CAD build for the part. Positions are in the model's coordinates, mm. A direction names the side the tool comes from. Round coordinates to 2 decimals unless told otherwise and drop trailing zeros. Write each loop counter-clockwise with the first axis right and the second up, starting at its lowest first coordinate (ties: lowest second). Pieces come first, ordered by that corner, then holes. Notation, with made-up numbers: (37, 3) - (92, 3) arc R29 cw to (92, 30) - close; hole circle Ø7 at (-20.75, 28). An arc over 180 degrees is marked (long way). Put each result on its own line as item: value. Start each with the question number.
Item 1: Cut at A-A (x = 13). Give the cut face in (y, z).
Item 2: Cut at D-D (x = 32.9). Give the cut face in (y, z), and give its area (3 significant figures).
Item 3: 3-axis set-ups, long thin cutter, end or side, ignore diameter. For faces 1 (the cylindrical face through (-16.5, 19.13, 2.54)), 2 (the cylindrical face through (-15.95, 15.7, 3.03)): which of +Z, -Z, +X, -X, +Y, -Y reach the whole face in a straight line?
Item 4: Drill centre lines: line 1 (Y direction, x = 13, z = 3.65); line 2 (Y direction, x = 13, z = 0.35); line 3 (Y direction, x = -12.1, z = 2.5). Where is each one in solid material? Low to high. Write a range as from..to.
Item 5: Mould opens along Y. For faces 3 (the cylindrical face through (102.3, 19.13, 2.54)), 4 (the flat face through (15, 11, 1)), 5 (the flat face through (30, 5, 0)) say: released by +Y, released by -Y, zero draft, split by the parting line, or undercut.
Item 6: Pin check, flat tip, straight feed: pin 1 Ø6.5 at (x, y) = (-11, 14) entering from +Z. Stop position of the tip, or through.
Item 7: Cut at C-C (y = -13). Give the cut face in (x, z), and give its area (3 significant figures).
Item 8: Cut at B-B (z = 3.5). Count the separate pieces of the cut face and the enclosed holes in it, and give its area (3 significant figures).
```python
from build123d import *

# Parameters (mm, degrees)
BOSS_EXTRUDE1_DEPTH            = 5
CBORE_FOR_M4_SHCS1_D           = 4.3
CBORE_FOR_M4_SHCS1_CBORE_D     = 8
CBORE_FOR_M4_SHCS1_CBORE_DEPTH = 4
M4_CLEARANCE_HOLE1_D           = 4.3
TAP_DRILL_FOR_M3X0_5_TAP1_D    = 2.5
M3_CLEARANCE_HOLE2_D           = 3.2
FILLET1_R                      = 2


with BuildPart() as part:
    # Sketch1 → Boss-Extrude1 (new body)
    with BuildSketch(Plane.XY):
        Polygon((17.1, 19.7), (102.9, 19.7), (102.9, 9.7), (17.1, -19.7), (-17.1, -19.7), (-17.1, 19.7), align=None)
    extrude(amount=BOSS_EXTRUDE1_DEPTH)

    # CBORE for M4 SHCS1 (through all)
    with Locations(Plane.XY.offset(5)):
        with Locations((13, 13), (-13, 13)):
            CounterBoreHole(CBORE_FOR_M4_SHCS1_D / 2, CBORE_FOR_M4_SHCS1_CBORE_D / 2, CBORE_FOR_M4_SHCS1_CBORE_DEPTH)

    # M4 Clearance Hole1 (through all)
    with Locations(Plane.XY.offset(5)):
        with Locations((-13, -13), (13, -13)):
            Hole(M4_CLEARANCE_HOLE1_D / 2)

    # Tap Drill for M3x0.5 Tap1 (through all)
    with Locations(Plane.XY.offset(5)):
        with Locations((-12.1, 3.8), (17.9, 3.8)):
            Hole(TAP_DRILL_FOR_M3X0_5_TAP1_D / 2)

    # M3 Clearance Hole2 (through all)
    with Locations(Plane(origin=(0, 0, 0), x_dir=(-1, 0, 0), z_dir=(0, 0, -1))):
        with Locations((-97.9, 14.7), (-32.9, 14.7)):
            Hole(M3_CLEARANCE_HOLE2_D / 2)

    # Fillet1
    fillet1_edges = [part.edges().sort_by_distance(p)[0] for p in [
        (-17.1, 19.7, 2.5),
        (102.9, 19.7, 2.5),
        (102.9, 9.7, 2.5),
        (17.1, -19.7, 2.5),
        (-17.1, -19.7, 2.5),
    ]]
    fillet(fillet1_edges, radius=FILLET1_R)


solid = part.part
```
Output values:
1. outline: (-19.7, 0) - (-15.15, 0) - (-15.15, 5) - (-19.7, 5) - close; (-10.85, 0) - (10.85, 0) - (10.85, 1) - (9, 1) - (9, 5) - (-10.85, 5) - close; (15.15, 0) - (19.7, 0) - (19.7, 5) - (17, 5) - (17, 1) - (15.15, 1) - close
2. outline: (-14.29, 0) - (13.1, 0) - (13.1, 5) - (-14.29, 5) - close; (16.3, 0) - (19.7, 0) - (19.7, 5) - (16.3, 5) - close
2. area: 154 mm2
3. face 1: +Z, -Z, -X, +Y
3. face 2: +Z
4. line 1: -19.7..-15.15, -10.85..9, 17..19.7
4. line 2: -19.7..-15.15, -10.85..10.85, 15.15..19.7
4. line 3: -19.7..-14.95, -11.05..2.55, 5.05..9.1, 16.9..19.7
5. face 3: released by +Y
5. face 4: undercut
5. face 5: zero draft
6. pin 1: z = 5
7. outline: (-17.1, 0) - (-15.15, 0) - (-15.15, 5) - (-17.1, 5) - close; (-10.85, 0) - (10.85, 0) - (10.85, 5) - (-10.85, 5) - close; (15.15, 0) - (36.65, 0) - (36.65, 5) - (15.15, 5) - close
7. area: 226 mm2
8. separate pieces: 1
8. enclosed holes: 8
8. area: 3,310 mm2
